Check sheet for the modelled part. Datum: model origin and axes. Units: mm. A direction names the side the tool comes from. Give positions to 0.01 mm unless a question says otherwise; leave off trailing zeros. Loops run counter-clockwise (first coordinate to the right, second up) from the corner with the lowest first, then second, coordinate; pieces in that order, holes last. Notation, with made-up numbers: (10, 24) - (23, 24) arc R22 ccw to (23, 32) - close; hole circle Ø7 at (15.25, -38). An arc over 180 degrees is marked (long way). Use CSV: the item, a comma, the result in double quotes.
from build123d import *

# Parameters (mm, degrees)
SKETCH1_W               = 50
SKETCH1_H               = 150
BOSS_EXTRUDE1_DEPTH     = 55
CUT_EXTRUDE1_DEPTH      = 168.406690428
CUT_EXTRUDE1_DEPTH_BACK = 45
SKETCH2_R               = 10.25
SKETCH7_R               = 1
SKETCH7_R_2             = 4.25
CUT_EXTRUDE3_DEPTH      = 10
BOSS_EXTRUDE2_START     = 45
SKETCH8_R               = 10.25
SKETCH8_R_2             = 1
SKETCH8_R_3             = 4.25
BOSS_EXTRUDE2_DEPTH     = 45
SKETCH9_R               = 10.25
CUT_EXTRUDE4_DEPTH      = 45


with BuildPart() as part:
    # Sketch1 → Boss-Extrude1 (new body)
    with BuildSketch(Plane.XY):
        with Locations((0, -75)):
            Rectangle(SKETCH1_W, SKETCH1_H)
    extrude(amount=-BOSS_EXTRUDE1_DEPTH)

    # Sketch2 → Cut-Extrude1 (cut, two sides: drawn at the far end of the back side and taken through both)
    with BuildSketch(Plane(origin=(25, 0, 0), x_dir=(0, 0, -1), z_dir=(1, 0, 0)).offset(-CUT_EXTRUDE1_DEPTH_BACK)):
        with Locations(Location((27.5, -25, 0), (0, 0, 270))):
            Circle(SKETCH2_R)
    extrude(amount=CUT_EXTRUDE1_DEPTH + CUT_EXTRUDE1_DEPTH_BACK, mode=Mode.SUBTRACT)

    # Sketch7 → Cut-Extrude3 (cut)
    with BuildSketch(Plane(origin=(-20, 0, 0), x_dir=(0, 0, -1), z_dir=(1, 0, 0))):
        with Locations(Location((27.5, -17, 0), (0, 0, 90))):
            Circle(SKETCH7_R)
        with Locations(Location((35.5, -25, 0), (0, 0, 90))):
            Circle(SKETCH7_R)
        with Locations(Location((27.5, -33, 0), (0, 0, 90))):
            Circle(SKETCH7_R)
        with Locations(Location((19.5, -25, 0), (0, 0, 90))):
            Circle(SKETCH7_R)
        with Locations(Location((27.5, -25, 0), (0, 0, 90))):
            Circle(SKETCH7_R_2)
    extrude(amount=-CUT_EXTRUDE3_DEPTH, mode=Mode.SUBTRACT)

    # Sketch8 → Boss-Extrude2 (add)
    with BuildSketch(Plane(origin=(-20, 0, 0), x_dir=(0, 0, -1), z_dir=(1, 0, 0)).offset(BOSS_EXTRUDE2_START)):
        with Locations((27.5, -25)):
            Circle(SKETCH8_R)
        with Locations(Location((27.5, -17, 0), (0, 0, 90))):
            Circle(SKETCH8_R_2, mode=Mode.SUBTRACT)
        with Locations(Location((27.5, -25, 0), (0, 0, 90))):
            Circle(SKETCH8_R_3, mode=Mode.SUBTRACT)
        with Locations(Location((35.5, -25, 0), (0, 0, 90))):
            Circle(SKETCH8_R_2, mode=Mode.SUBTRACT)
        with Locations(Location((27.5, -33, 0), (0, 0, 90))):
            Circle(SKETCH8_R_2, mode=Mode.SUBTRACT)
        with Locations(Location((19.5, -25, 0), (0, 0, 90))):
            Circle(SKETCH8_R_2, mode=Mode.SUBTRACT)
    extrude(amount=-BOSS_EXTRUDE2_DEPTH)

    # Sketch9 → Cut-Extrude4 (cut)
    with BuildSketch(Plane.ZY.offset(25)):
        with Locations(Location((-27.5, -25, 0), (0, 0, 270))):
            Circle(SKETCH9_R)
    extrude(amount=-CUT_EXTRUDE4_DEPTH, mode=Mode.SUBTRACT)


solid = part.part
1. Scan lines: line 1 along Z through (x, y) = (21.75, -25); line 2 along Z through (x, y) = (-5, -25); line 3 along Z through (x, y) = (22.15, -33). Record each from-to range of solid material in increasing order.
Completed:
line 1,"z = -55 to -36.5, -34.5 to -31.75, -23.25 to -20.5, -18.5 to 0"
line 2,"z = -55 to -37.75, -17.25 to 0"
line 3,"z = -55 to -28.5, -26.5 to 0"
2. Set-up check for faces 1 (the face through (20, -29.4, -27.4)), 2 (the face through (0, -74, 0)): record each of +Z, -Z, +X, -X, +Y, -Y from which the full face is reachable in a straight line by a thin tool's end or side.
Completed:
face 1,"-X"
face 2,"+Z, +X, -X, +Y, -Y"
3. Go/stop test with flat-tipped pins: pin 1 Ø6 at (x, z) = (8.5, -42.5) entering from +Y; pin 2 Ø2.5 at (y, z) = (-33, -27.5) entering from -X. Record where each tip stops, or that it passes through.
Completed:
pin 1,"stops at y = 0"
pin 2,"stops at x = 20"
4. Sectioned sample at A-A, the plane x = -10. Record the boundary of the cut face in (y, z), and give its area (3 significant figures).
Completed:
outline,"(-150, -55) - (0, -55) - (0, 0) - (-150, 0) - close; hole circle Ø20.5 at (-25, -27.5)"
area,"7,920 mm²"
5. Release check for a two-part mould opening along Y. For faces 3 (the face through (0, 0, -27)), 4 (the face through (-25, -76, -27)), 5 (the face through (22.54, -28.37, -30.09)) record: released by +Y, released by -Y, zero draft, split by the parting line, or undercut.
Completed:
face 3,"released by +Y"
face 4,"zero draft"
face 5,"undercut"
